from build123d import *

# Parameters (mm, degrees)
SKETCH1_W           = 63.5
SKETCH1_H           = 38.1
BOSS_EXTRUDE1_DEPTH = 12.7


with BuildPart() as part:
    # Sketch1 → Boss-Extrude1 (new body)
    with BuildSketch(Plane(origin=(0, 0, 0), x_dir=(1, 0, 0), z_dir=(0, 1, 0))):
        Rectangle(SKETCH1_W, SKETCH1_H)
    extrude(amount=BOSS_EXTRUDE1_DEPTH)

    # Sketch5 → #10-32 Tapped Hole1 (revolve, cut)
    with BuildSketch(Plane(origin=(-31.75, 6.35, 0), x_dir=(0, 0, 1), z_dir=(0, 1, 0))):
        Polygon((0, 0), (0, 13.151317848), (2.0193, 11.938), (2.0193, 0), align=None)
    f_10_32_tapped_hole1 = revolve(axis=Axis((-38.1, 6.35, 0), (1, 0, 0)), mode=Mode.SUBTRACT)

    # Mirror1: #10-32 Tapped Hole1 across plane
    add(f_10_32_tapped_hole1.mirror(Plane(origin=(0, 0, 0), x_dir=(0, 0, 1), z_dir=(1, 0, 0))), mode=Mode.SUBTRACT)


solid = part.part
Could you check a few things on this model? Use its own coordinates, in mm. A direction names the side the tool comes from. Coordinates: 2 decimals unless noted, no trailing zeros. Write each loop counter-clockwise with the first axis right and the second up, starting at its lowest first coordinate (ties: lowest second). Pieces come first, ordered by that corner, then holes. Notation, with made-up numbers: (-19.5, 16.25) - (16.5, 16.25) arc R4 ccw to (16.5, 21.25) - close; hole circle Ø8 at (-36, 78). An arc over 180 degrees is marked (long way). Put each result on its own line as item: value. Start each with the question number.
Q1. Please list where these lines run through material, in increasing order: L1, parallel to Y at x = -24, z = 0; L2, parallel to Z at x = -29, y = 6.35; L3, parallel to Z at x = -27.5, y = 5.5.
Q2. Thinking about a two-plate mould opening in Z: for faces 3 (the flat face through (0, 6, 19.05)), 4 (the flat face through (0, 0, 0)), 5 (the cylindrical face through (25.865, 4.348, -0.263)), 6 (the conical face through (-18.81, 6.66, 0.16)), which applies, pulls with the +Z half, pulls with the -Z half, needs draft (parallel to the pull), parting line crosses it, or undercut?
Q3. I want a section at A-A on x = -24.5. Write out the boundary of the cut face in (y, z), plus the area to 3 significant figures.
Q4. Which directions (+Z, -Z, +X, -X, +Y, -Y) give clear straight access to the entire face, cutting with the end or side of a thin tool? Please do faces 1 (the flat face through (0, 12.7, 0)), 2 (the cylindrical face through (-25.865, 4.348, -0.263)).
Q5. I'm going to push a flat-ended pin straight in: P1, Ø3.5, axis at y = 6.35, z = 0, coming from the -X side. Where does the tip first touch, or does it pass through?
Checks:
1. L1: 0 to 4.33, 8.37 to 12.7
1. L2: -19.05 to -2.02, 2.02 to 19.05
1. L3: -19.05 to -1.83, 1.83 to 19.05
2. face 3: pulls with the +Z half
2. face 4: needs draft
2. face 5: undercut
2. face 6: undercut
3. outline: (0, -19.05) - (12.7, -19.05) - (12.7, 19.05) - (0, 19.05) - close; hole circle Ø4.04 at (6.35, 0)
3. area: 471 mm²
4. face 1: +Z, -Z, +X, -X, +Y
4. face 2: -X
5. P1: x = -19.65
